Autodesk Inventor part; units mm, degrees
ref_plane "YZ Plane" through (0, 0, 0) normal (1, 0, 0) x (0, 1, 0)
ref_plane "XZ Plane" through (0, 0, 0) normal (0, 1, 0) x (-1, 0, 0)
ref_plane "XY Plane" through (0, 0, 0) normal (0, 0, 1) x (1, 0, 0)
sketch "Sketch1" plane through (0, 0, 0) normal (0, 0, 1) x (1, 0, 0)
  line L0 (-50, 45) -> (50, 45)
  line L1 (50, 45) -> (50, 40)
  line L2 (50, 40) -> (21, -40)
  line L3 (21, -40) -> (21, -50)
  line L4 (21, -50) -> (-21, -50)
  line L5 (-21, -50) -> (-21, -40)
  line L6 (-21, -40) -> (-50, 40)
  line L7 (-50, 40) -> (-50, 45)
  point P0 (0, 0)
  point P1 (0, -50)
  point P2 (0, 45)
  point P3 (-35.5, 0)
  dimension "d0" = 42
  dimension "d1" = 10
  dimension "d2" = 5
  dimension "d3" = 95
  dimension "d4" = 100
extrude "Extrusion1" add sketch "Sketch1" along normal blind 20
sketch "Sketch2" plane through (-21, -50, 0) normal (0, -1, 0) x (1, 0, 0)
  line L0 (0, 20) -> (42, 20)
  line L1 (0, 0) -> (0, 20)
  line L2 (0, 20) -> (42, 20)
  line L3 (42, 20) -> (42, 62)
  line L4 (42, 62) -> (0, 62)
  line L5 (0, 62) -> (0, 20)
  circle A0 centre (21, 41) radius 11.25
  circle A1 centre (5.5, 56.5) radius 1.75
  circle A2 centre (5.5, 25.5) radius 1.75
  circle A3 centre (36.5, 25.5) radius 1.75
  circle A4 centre (36.5, 56.5) radius 1.75
  point P0 (21, 0)
  point P1 (21, 62)
  point P2 (0, 41)
  dimension "d7" = 22.5
  dimension "d8" = 31
  dimension "d9" = 31
  dimension "d10" = 15.5
  dimension "d11" = 15.5
  dimension "d12" = 3.5
extrude "Extrusion2" add sketch "Sketch2" against normal blind 10
sketch "Sketch3" plane through (-21, -50, 0) normal (0, -1, 0) x (1, 0, 0)
  line L0 (71, 0) -> (-29, 0)
  line L1 (-29, 0) -> (-29, 20)
  line L2 (71, 20) -> (-29, 20)
  line L3 (71, 0) -> (71, 20)
  circle A0 centre (-17, 10) radius 5
  circle A1 centre (-17, 10) radius 2.15
  circle A2 centre (59, 10) radius 5
  circle A3 centre (59, 10) radius 2.15
  circle A4 centre (10, 10) radius 5
  circle A5 centre (32, 10) radius 5
  circle A6 centre (32, 10) radius 2.15
  circle A7 centre (10, 10) radius 2.15
  line L4 (0, 0) -> (0, 62)
  line L5 (42, 0) -> (42, 62)
  point P0 (21, 0)
  point P1 (-29, 10)
  dimension "d15" = 12
  dimension "d16" = 4.3
  dimension "d17" = 10
  dimension "d18" = 12
  dimension "d19" = 10
  dimension "d20" = 10
extrude "Extrusion3" cut sketch "Sketch3" against normal blind 92 contours A0 | A1 | A2 | A3 | A4 | A5 | A6 | A7
extrude "Extrusion5" cut sketch "Sketch3" against normal through all contours A1 | A3 | A6 | A7
sketch "Sketch4" plane through (0, 0, 20) normal (0, 0, 1) x (1, 0, 0)
  circle A0 centre (0, 40) radius 2.1
  circle A1 centre (0, 10) radius 2.1
  circle A2 centre (0, -20) radius 2.1
  line L0 (50, 45) -> (-50, 45)
  point P0 (0, 0)
  dimension "d23" = 5
  dimension "d24" = 30
  dimension "d25" = 30
  dimension "d26" = 4.2
extrude "Extrusion4" cut sketch "Sketch4" against normal blind 10
equation "\"d9\" = d8"
equation "\"d10\" = 0.5 * d8"
equation "\"d11\" = 0.5 * d9"
equation "\"d18\" = d15"
equation "\"d20\" = d19"
properties part number "SliderMotorHalter"
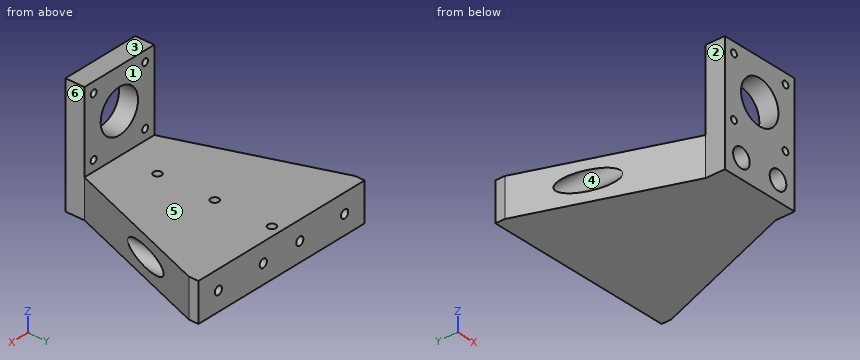
Read the model definition and answer for the solid it produces. Units are mm, in the model's axes. Face numbers are marked on the shaded views. A direction names the side the tool comes from. Round coordinates to 2 decimals unless told otherwise and drop trailing zeros. Order: outer loops, then holes, each group sorted by start corner. A loop starts at its lowest first (then second) coordinate and runs counter-clockwise, first axis right, second up.
1) The part is cut by section D-D on z = 49. Write down the section's boundary in (x, y), plus the area to 3 significant figures.
2) The mould has two halves that part along X. Classify the marked faces 4, 5 and 6: released by +X, released by -X, zero draft, split by the parting line, or undercut.
3) Flat-ended cylindrical pins translate along their axes: pin 1 (6.5 mm diameter, centred on x = 0, y = 10, fed in from -Z); pin 2 (3.5 mm diameter, centred on x = -11, z = 10, fed in from -Y) (3 decimals); pin 3 (3 mm diameter, centred on y = -38.5, z = 14, fed in from +X); pin 4 (3 mm diameter, centred on x = -39.5, z = 7.5, fed in from -Y). Find the tip coordinate at first contact, or state that the pin passes through.
4) Straight lines are drawn through the part: L1, parallel to Z at x = -15.5, y = -48; L2, parallel to Y at x = 0, z = 17; L3, parallel to Z at x = 11, y = 43. For each, find the intervals that lie inside material, in ascending order.
5) The part is cut by section B-B on z = 56.5. Write down the section's boundary in (x, y).
6) The part is cut by section A-A on y = -43. Write down the section's boundary in (x, z), plus the area to 3 significant figures.
7) The part is cut by section C-C on y = -20. Write down the section's boundary in (x, z), plus the area to 3 significant figures.
8) For the marked faces 1, 2 and 3, determine the directions among +Z, -Z, +X, -X, +Y, -Y from which every point of the face is accessible in a straight line to the end or side of a thin tool.
Resolved:
1. outline: (-21, -50) - (-7.91, -50) - (-7.91, -40) - (-21, -40) - close; (7.91, -50) - (21, -50) - (21, -40) - (7.91, -40) - close
1. area: 262 mm2
2. face 4: undercut
2. face 5: zero draft
2. face 6: released by +X
3. pin 1: stops at z = 0
3. pin 2: passes through
3. pin 3: stops at x = 22.09
3. pin 4: stops at y = 42
4. L1: z = 0 to 7.82, 12.18 to 23.75, 27.25 to 54.75, 58.25 to 62
4. L2: y = -50 to -22.1, -17.9 to 7.9, 12.1 to 37.9, 42.1 to 45
4. L3: z = 0 to 7.85, 12.15 to 20
5. outline: (-21, -50) - (-17.25, -50) - (-17.25, -40) - (-21, -40) - close; (-13.75, -50) - (13.75, -50) - (13.75, -40) - (-13.75, -40) - close; (17.25, -50) - (21, -50) - (21, -40) - (17.25, -40) - close
6. outline: (-21, 0) - (21, 0) - (21, 62) - (-21, 62) - close; hole circle Ø3.5 at (-15.5, 25.5); hole circle Ø3.5 at (-15.5, 56.5); hole circle Ø10 at (-11, 10); hole circle Ø22.5 at (0, 41); hole circle Ø10 at (11, 10); hole circle Ø3.5 at (15.5, 25.5); hole circle Ø3.5 at (15.5, 56.5)
6. area: 2,010 mm2
7. outline: (-28.25, 0) - (28.25, 0) - (28.25, 20) - (2.1, 20) - (2.1, 10) - (-2.1, 10) - (-2.1, 20) - (-28.25, 20) - close; hole circle Ø10 at (-11, 10); hole circle Ø10 at (11, 10)
7. area: 931 mm2
8. face 1: +Z, +X, -X, +Y
8. face 2: +Z, -Z, -X, -Y
8. face 3: +Z, +X, -X, +Y, -Y
